Can you work these out from the model? Positions are in its coordinate system, mm. A direction names the side the tool comes from. Coordinates: 2 decimals unless noted, no trailing zeros. Write each loop counter-clockwise with the first axis right and the second up, starting at its lowest first coordinate (ties: lowest second). Pieces come first, ordered by that corner, then holes. Notation, with made-up numbers: (33, -38) - (74, -38) arc R16 cw to (74, -17) - close; hole circle Ø8 at (35, 51). An arc over 180 degrees is marked (long way). Write each question's results on one line, items separated by ' | '. Start each with the question number.
```python
from build123d import *

# Parameters (mm, degrees)
F2_DEPTH     = 25.4
F3_R         = 5.08
F4_T1_DEPTH  = 63.7089962256
F4_T3_DEPTH  = 34.3299805756
F4_T5_DEPTH  = 39.8420593032
F4_T7_DEPTH  = 15.24
F4_T12_DEPTH = 5.08
F4_T18_DEPTH = 5.08
F4_T24_DEPTH = 5.08
F4_T30_DEPTH = 5.08
F4_T36_DEPTH = 37.6403571065
F4_T41_DEPTH = 43.8944483223
F4_T46_DEPTH = 48.4484626095
F4_T51_DEPTH = 34.2442917913
F4_T57_DEPTH = 43.8944483223
F4_T61_DEPTH = 37.6403571065
F4_T68_DEPTH = 48.4484626095
F4_T72_DEPTH = 34.2442917913


# Not quite as in the source:
# - a fillet or chamfer that OpenCascade refuses, or shapes differently, is made with other operations: its cross-section is extruded or revolved along the edge and cut away or added


with BuildPart() as f2:
    # F1 (on face) → F2 (new body)
    with BuildSketch(Plane.XY):
        Polygon((8.4329312667, 10.7982652262), (-6.5817977302, 0), (-37.6396663487, 0), (-35.5828553438, -11.0039459541), (-30.0294607878, -17.1743836254), (23.241976276, -17.1743836254), (31.0578662902, -12.8550762311), (37.6396663487, 0), (28.7953745574, 0), align=None)
    extrude(amount=F2_DEPTH)

    # F3
    f3_edges = [f2.edges().sort_by_distance(p)[0] for p in [
        (-22.110732, 0, 25.4),
        (18.614153, 5.399133, 25.4),
        (33.21752, 0, 25.4),
        (34.348766, -6.427538, 25.4),
        (27.149921, -15.01473, 25.4),
        (-3.393742, -17.174384, 25.4),
        (-32.806158, -14.089165, 25.4),
        (-36.611261, -5.501973, 25.4),
        (-32.806158, -14.089165, 0),
        (-36.611261, -5.501973, 0),
        (-35.582855, -11.003946, 12.7),
        (0.925567, 5.399133, 25.4),
    ]]
    fillet(f3_edges, radius=F3_R)

    # F4: fillet of radius 5.08 on 11 edges, made by hand

    # F4_s2 → F4_t1 (cut)
    with BuildSketch(Plane.YZ.offset(-27.7670199495)):
        with BuildLine():
            ThreePointArc((-12.0943836254, 0), (-15.6864860738, 1.4878975516), (-17.1743836254, 5.08))
            Line((-17.1743836254, 5.08), (-17.1743836254, 0))
            Line((-17.1743836254, 0), (-12.0943836254, 0))
        make_face()
    extrude(amount=F4_T1_DEPTH, mode=Mode.SUBTRACT)

    # F4_s4 → F4_t3 (cut)
    with BuildSketch(Plane(origin=(-0.5817443509, -0.3214902809, 0), x_dir=(0, 0, 1), z_dir=(0.8752415471, 0.4836860907, 0))):
        with BuildLine():
            ThreePointArc((0, 21.1935547384), (1.4878975516, 24.7856571868), (5.08, 26.2735547384))
            Line((5.08, 26.2735547384), (0, 26.2735547384))
            Line((0, 26.2735547384), (0, 21.1935547384))
        make_face()
    extrude(amount=F4_T3_DEPTH, mode=Mode.SUBTRACT)

    # F4_s6 → F4_t5 (cut)
    with BuildSketch(Plane(origin=(-4.5520149502, -8.8906528107, 0), x_dir=(0, 0, 1), z_dir=(0.4557383348, 0.8901137962, 0))):
        with BuildLine():
            ThreePointArc((0, 28.4235863007), (1.4878975516, 32.0156887492), (5.08, 33.5035863007))
            Line((5.08, 33.5035863007), (0, 33.5035863007))
            Line((0, 33.5035863007), (0, 28.4235863007))
        make_face()
    extrude(amount=F4_T5_DEPTH, mode=Mode.SUBTRACT)

    # F4_s8 → F4_t7 (cut)
    with BuildSketch(Plane.XY.offset(5.08)):
        with BuildLine():
            ThreePointArc((-31.5221548367, 0), (-35.430345336, -1.8346268287), (-36.5156731811, -6.0133673145))
            Line((-36.5156731811, -6.0133673145), (-37.6396663487, 0))
            Line((-37.6396663487, 0), (-31.5221548367, 0))
        make_face()
        with BuildLine():
            ThreePointArc((-27.7670199495, -17.1743836254), (-29.8337598255, -16.7349640077), (-31.5429540141, -15.4927246824))
            Line((-31.5429540141, -15.4927246824), (-30.0294607878, -17.1743836254))
            Line((-30.0294607878, -17.1743836254), (-27.7670199495, -17.1743836254))
        make_face()
    extrude(amount=F4_T7_DEPTH, mode=Mode.SUBTRACT)


with BuildPart() as f4_tool10:
    # F4_s11 → F4_t12 (new body)
    with BuildSketch(Plane.XY.offset(20.32)):
        Polygon((-27.7670199495, -12.0943836254), (-27.7670199495, -17.1743836254), (-30.0294607878, -17.1743836254), (-31.5429540141, -15.4927246824), align=None)
    extrude(amount=F4_T12_DEPTH)

    # F4_s13 → F4_t14 (revolve, cut)
    with BuildSketch(Plane(origin=(-27.7670199495, -12.0943836254, 20.32), x_dir=(0.4068385583, 0.9135000753, 0), z_dir=(0.9135000753, -0.4068385583, 0))):
        with BuildLine():
            ThreePointArc((0, -5.08), (5.08, 0), (0, 5.08))
            Line((0, 5.08), (0, -5.08))
        make_face()
    revolve(axis=Axis((-27.7670199495, -12.0943836254, 20.32), (0, 0, 1)), mode=Mode.SUBTRACT)


with BuildPart() as f2_1:
    add(f2.part)

    # F4_t9: cut F4_tool10
    add(f4_tool10.part, mode=Mode.SUBTRACT)


with BuildPart() as f4_tool16:
    # F4_s17 → F4_t18 (new body)
    with BuildSketch(Plane.XY.offset(20.32)):
        Polygon((-31.5221548367, -5.08), (-31.5221548367, 0), (-37.6396663487, 0), (-36.5156731811, -6.0133673145), align=None)
    extrude(amount=F4_T18_DEPTH)

    # F4_s19 → F4_t20 (revolve, cut)
    with BuildSketch(Plane(origin=(-31.5221548367, -5.08, 20.32), x_dir=(0.7693288384, -0.6388529865, 0), z_dir=(-0.6388529865, -0.7693288384, 0))):
        with BuildLine():
            ThreePointArc((0, -5.08), (5.08, 0), (0, 5.08))
            Line((0, 5.08), (0, -5.08))
        make_face()
    revolve(axis=Axis((-31.5221548367, -5.08, 20.32), (0, 0, 1)), mode=Mode.SUBTRACT)


with BuildPart() as f2_2:
    add(f2_1.part)

    # F4_t15: cut F4_tool16
    add(f4_tool16.part, mode=Mode.SUBTRACT)


with BuildPart() as f4_tool22:
    # F4_s23 → F4_t24 (new body)
    with BuildSketch(Plane.XY.offset(5.08)):
        Polygon((-27.7670199495, -12.0943836254), (-27.7670199495, -17.1743836254), (-30.0294607878, -17.1743836254), (-31.5429540141, -15.4927246824), align=None)
    extrude(amount=-F4_T24_DEPTH)

    # F4_s25 → F4_t26 (revolve, cut)
    with BuildSketch(Plane(origin=(-27.7670199495, -12.0943836254, 5.08), x_dir=(0.4068385583, 0.9135000753, 0), z_dir=(-0.9135000753, 0.4068385583, 0))):
        with BuildLine():
            ThreePointArc((0, -5.08), (5.08, 0), (0, 5.08))
            Line((0, 5.08), (0, -5.08))
        make_face()
    revolve(axis=Axis((-27.7670199495, -12.0943836254, 5.08), (0, 0, -1)), mode=Mode.SUBTRACT)


with BuildPart() as f2_3:
    add(f2_2.part)

    # F4_t21: cut F4_tool22
    add(f4_tool22.part, mode=Mode.SUBTRACT)


with BuildPart() as f4_tool28:
    # F4_s29 → F4_t30 (new body)
    with BuildSketch(Plane.XY.offset(5.08)):
        Polygon((-31.5221548367, -5.08), (-31.5221548367, 0), (-37.6396663487, 0), (-36.5156731811, -6.0133673145), align=None)
    extrude(amount=-F4_T30_DEPTH)

    # F4_s31 → F4_t32 (revolve, cut)
    with BuildSketch(Plane(origin=(-31.5221548367, -5.08, 5.08), x_dir=(0.7693288384, -0.6388529865, 0), z_dir=(0.6388529865, 0.7693288384, 0))):
        with BuildLine():
            ThreePointArc((0, -5.08), (5.08, 0), (0, 5.08))
            Line((0, 5.08), (0, -5.08))
        make_face()
    revolve(axis=Axis((-31.5221548367, -5.08, 5.08), (0, 0, -1)), mode=Mode.SUBTRACT)


with BuildPart() as f2_4:
    add(f2_3.part)

    # F4_t27: cut F4_tool28
    add(f4_tool28.part, mode=Mode.SUBTRACT)


with BuildPart() as f4_tool34:
    # F4_s35 → F4_t36 (new body)
    with BuildSketch(Plane.YZ.offset(6.1182022698)):
        with BuildLine():
            ThreePointArc((-5.08, 0), (-1.4878975516, 1.4878975516), (0, 5.08))
            Line((0, 5.08), (0, 0))
            Line((0, 0), (-5.08, 0))
        make_face()
    extrude(amount=-F4_T36_DEPTH)

    split(bisect_by=Plane(origin=(-2.2437256361, 3.119846722, 0), x_dir=(0, 0, 1), z_dir=(-0.5838652247, 0.8118506016, 0)), keep=Keep.TOP)


with BuildPart() as f2_5:
    add(f2_4.part)

    # F4_t33: cut F4_tool34
    add(f4_tool34.part, mode=Mode.SUBTRACT)


with BuildPart() as f4_tool39:
    # F4_s40 → F4_t41 (new body)
    with BuildSketch(Plane(origin=(20.9871595433, 15.0935068584, 0), x_dir=(0, 0, 1), z_dir=(-0.8118506016, -0.5838652247, 0))):
        with BuildLine():
            ThreePointArc((5.08, 3.8428828109), (1.4878975516, 2.3549852594), (0, -1.2371171891))
            Line((0, -1.2371171891), (0, 3.8428828109))
            Line((0, 3.8428828109), (5.08, 3.8428828109))
        make_face()
    extrude(amount=F4_T41_DEPTH)

    split(bisect_by=Plane.XZ, keep=Keep.BOTTOM)


with BuildPart() as f2_6:
    add(f2_5.part)

    # F4_t38: cut F4_tool39
    add(f4_tool39.part, mode=Mode.SUBTRACT)


with BuildPart() as f4_tool44:
    # F4_s45 → F4_t46 (new body)
    with BuildSketch(Plane(origin=(33.6949109219, -17.8685131108, 0), x_dir=(0, 0, 1), z_dir=(-0.8834621049, 0.4685026246, 0))):
        with BuildLine():
            ThreePointArc((5.08, 13.4907085573), (1.4878975516, 12.0028110057), (0, 8.4107085573))
            Line((0, 8.4107085573), (0, 13.4907085573))
            Line((0, 13.4907085573), (5.08, 13.4907085573))
        make_face()
    extrude(amount=F4_T46_DEPTH)

    split(bisect_by=Plane.XZ, keep=Keep.BOTTOM)


with BuildPart() as f2_7:
    add(f2_6.part)

    # F4_t43: cut F4_tool44
    add(f4_tool44.part, mode=Mode.SUBTRACT)


with BuildPart() as f4_tool49:
    # F4_s50 → F4_t51 (new body)
    with BuildSketch(Plane.YZ.offset(50.3396663487)):
        with BuildLine():
            ThreePointArc((-5.08, 0), (-1.4878975516, 1.4878975516), (0, 5.08))
            Line((0, 5.08), (0, 0))
            Line((0, 0), (-5.08, 0))
        make_face()
    extrude(amount=-F4_T51_DEPTH)

    split(bisect_by=Plane(origin=(6.3204323672, 11.918529778, 0), x_dir=(0, 0, 1), z_dir=(0.4685026246, 0.8834621049, 0)), keep=Keep.TOP)


with BuildPart() as f2_8:
    add(f2_7.part)

    # F4_t48: cut F4_tool49
    add(f4_tool49.part, mode=Mode.SUBTRACT)


with BuildPart() as f4_tool55:
    # F4_s56 → F4_t57 (new body)
    with BuildSketch(Plane(origin=(20.9871595433, 15.0935068584, 0), x_dir=(0, 0, 1), z_dir=(-0.8118506016, -0.5838652247, 0))):
        with BuildLine():
            ThreePointArc((5.08, 3.8428828109), (1.4878975516, 2.3549852594), (0, -1.2371171891))
            Line((0, -1.2371171891), (0, 3.8428828109))
            Line((0, 3.8428828109), (5.08, 3.8428828109))
        make_face()
    extrude(amount=F4_T57_DEPTH)

    split(bisect_by=Plane.XZ, keep=Keep.TOP)


with BuildPart() as f4_tool59:
    # F4_s60 → F4_t61 (new body)
    with BuildSketch(Plane.YZ.offset(6.1182022698)):
        with BuildLine():
            ThreePointArc((-5.08, 0), (-1.4878975516, 1.4878975516), (0, 5.08))
            Line((0, 5.08), (0, 0))
            Line((0, 0), (-5.08, 0))
        make_face()
    extrude(amount=-F4_T61_DEPTH)

    split(bisect_by=Plane(origin=(-2.2437256361, 3.119846722, 0), x_dir=(0, 0, 1), z_dir=(0.5838652247, -0.8118506016, 0)), keep=Keep.TOP)


with BuildPart() as f4_tool55_1:
    add(f4_tool55.part)

    # F4_t63: intersect F4_tool59
    add(f4_tool59.part, mode=Mode.INTERSECT)


with BuildPart() as f2_9:
    add(f2_8.part)

    # F4_t53: cut F4_tool55
    add(f4_tool55_1.part, mode=Mode.SUBTRACT)


with BuildPart() as f4_tool66:
    # F4_s67 → F4_t68 (new body)
    with BuildSketch(Plane(origin=(33.6949109219, -17.8685131108, 0), x_dir=(0, 0, 1), z_dir=(-0.8834621049, 0.4685026246, 0))):
        with BuildLine():
            ThreePointArc((5.08, 13.4907085573), (1.4878975516, 12.0028110057), (0, 8.4107085573))
            Line((0, 8.4107085573), (0, 13.4907085573))
            Line((0, 13.4907085573), (5.08, 13.4907085573))
        make_face()
    extrude(amount=F4_T68_DEPTH)

    split(bisect_by=Plane.XZ, keep=Keep.TOP)


with BuildPart() as f4_tool70:
    # F4_s71 → F4_t72 (new body)
    with BuildSketch(Plane.YZ.offset(50.3396663487)):
        with BuildLine():
            ThreePointArc((-5.08, 0), (-1.4878975516, 1.4878975516), (0, 5.08))
            Line((0, 5.08), (0, 0))
            Line((0, 0), (-5.08, 0))
        make_face()
    extrude(amount=-F4_T72_DEPTH)

    split(bisect_by=Plane(origin=(6.3204323672, 11.918529778, 0), x_dir=(0, 0, 1), z_dir=(-0.4685026246, -0.8834621049, 0)), keep=Keep.TOP)


with BuildPart() as f4_tool66_1:
    add(f4_tool66.part)

    # F4_t74: intersect F4_tool70
    add(f4_tool70.part, mode=Mode.INTERSECT)


with BuildPart() as f2_10:
    add(f2_9.part)

    # F4_t64: cut F4_tool66
    add(f4_tool66_1.part, mode=Mode.SUBTRACT)


solid = f2_10.part
```
Q1. If we section it at A-A (x = -11.5): Please give me the cut outline in (y, z).
Q2. For faces 1 (the face through (33, 0, 13)), 2 (the face through (31.53, -0.95, 2.12)), 3 (the face through (-19, 0, 13)), 4 (the face through (-18.42, -1.449, 23.872)), 5 (the face through (32.51, -0.89, 23.19)), which set-ups out of +Z, -Z, +X, -X, +Y, -Y let a thin tool reach every point of the face, with its end or its side?
Q3. I need wall thicknesses on line 1 along Z through (x, y) = (20.5, -1); line 2 along Y through (x, z) = (-11.5, 8.5); line 3 along X through (y, z) = (-12.5, 12.25). Which ranges of each line are inside material? Lowest first, please. Write a range as from..to.
Q4. If we section it at B-B (z = 6): Please give me the cut outline in (x, y).
Q5. I'm going to push flat-ended pins straight in: pin 1 Ø1 at (y, z) = (-7.5, 13) entering from +X; pin 2 Ø8 at (y, z) = (-3, 21) entering from +X; pin 3 Ø4 at (y, z) = (1, 20.5) entering from -X; pin 4 Ø12 at (x, z) = (-13, 16.5) entering from +Y. Where does each tip first touch, or does it pass through?
Answer list:
1) outline: (-17.17, 5.08) arc R5.08 ccw to (-12.09, 0) - (-5.08, 0) arc R5.08 ccw to (0, 5.08) - (0, 20.32) arc R5.08 ccw to (-5.08, 25.4) - (-12.09, 25.4) arc R5.08 ccw to (-17.17, 20.32) - close
2) face 1: +Z, -Z, +X, +Y | face 2: -Z, +X, +Y | face 3: +Z, -Z, -X, +Y | face 4: +Z, -X, +Y | face 5: +Z, +X, +Y
3) line 1: z = 0.01..25.39 | line 2: y = -17.17..0 | line 3: x = -34.24..31.24
4) outline: (-36.52, -6.01) - (-35.85, -9.6) arc R5.08 ccw to (-34.63, -12.07) - (-31.54, -15.49) arc R5.08 ccw to (-27.77, -17.17) - (23.24, -17.17) - (31.06, -12.86) - (37.64, 0) - (28.8, 0) - (8.43, 10.8) - (-6.58, 0) - (-31.52, 0) arc R5.08 ccw to start
5) pin 1: stops at x = 34.06 | pin 2: stops at x = 37.64 | pin 3: stops at x = -34.55 | pin 4: stops at y = 0
